Geometry: see drawing. Coordinates: mm, zero at the bounding-box minimum. A direction names the side the tool comes from. Give positions to 0.01 mm unless a question says otherwise; leave off trailing zeros. Order: outer loops, then holes, each group sorted by start corner. A loop starts at its lowest first (then second) coordinate and runs counter-clockwise, first axis right, second up. Notation, with made-up numbers: (55, 38) - (111, 38) arc R18 ccw to (111, 72) - close; hole circle Ø1 at (39, -27.75). An arc over 180 degrees is marked (long way). Write item = value, one per line. Start each with the question number.
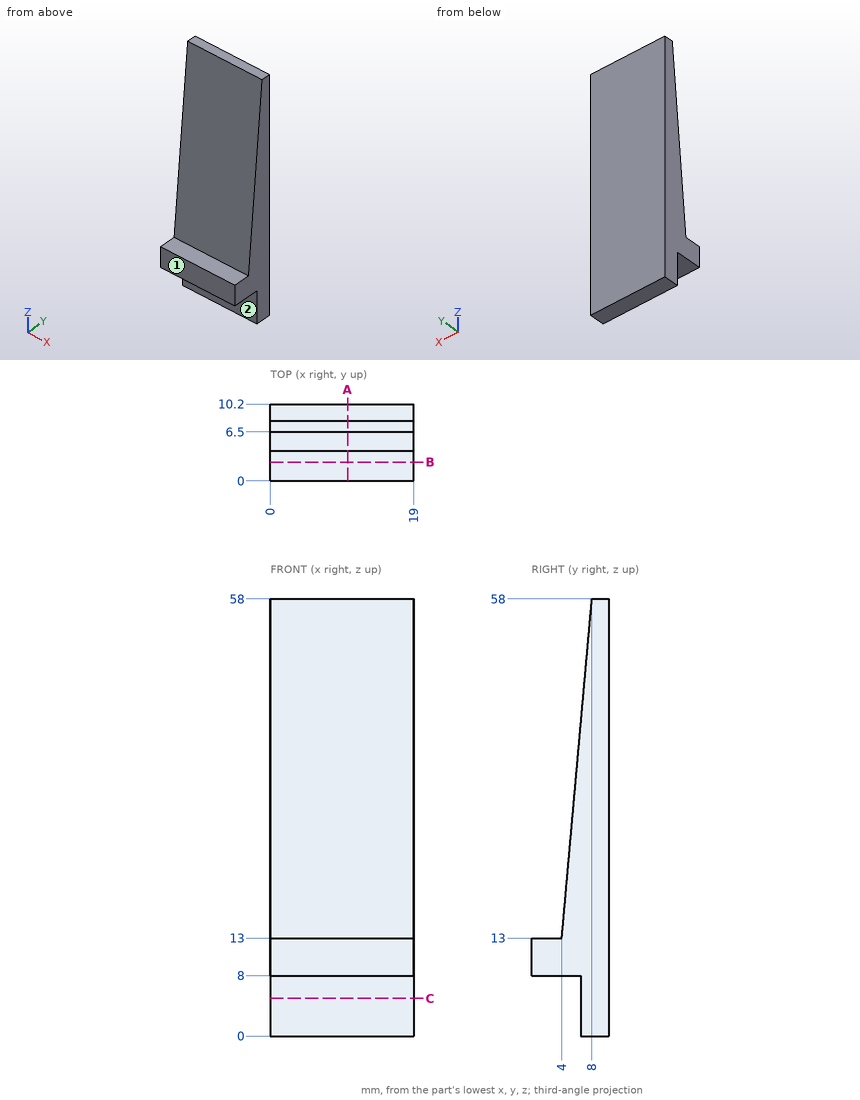
Q1. Material intervals for line 1 along Z through (x, y) = (13, 3.75); line 2 along Y through (x, z) = (2.25, 7); line 3 along Y through (x, z) = (7.25, 29.5), sorted ascending. Write a range as from..to.
Q2. Section A-A, the plane x = 10.25. Return the cut outline in (y, z).
Q3. Contact query for flat-ended pins moving along their axis: pin 1 (2 mm diameter, centred on y = 4, z = 39, fed in from -X); pin 2 (6 mm diameter, centred on x = 3.5, z = 42.5, fed in from -Y); pin 3 (4 mm diameter, centred on x = 6, z = 3.5, fed in from -Y); pin 4 (2 mm diameter, centred on x = 6, y = 2, fed in from +Z). Output: stop coordinate, or through.
Q4. Section B-B, the plane y = 2.5. Return the cut outline in (x, z), then the cut area to 3 significant figures.
Q5. Set-up query: the marked faces 1 and 2. Return all of +Z, -Z, +X, -X, +Y, -Y with unobstructed straight access to the full face (end or side cutting, diameter ignored); none if empty.
Q6. Section C-C, the plane z = 5. Return the cut outline in (x, y), then the cut area to 3 significant figures.
The answers:
q1.line_1 = 8..13
q1.line_2 = 6.5..10.2
q1.line_3 = 5.47..10.2
q2.outline = (0, 8) - (6.5, 8) - (6.5, 0) - (10.2, 0) - (10.2, 58) - (8, 58) - (4, 13) - (0, 13) - close
q3.pin_1 = through
q3.pin_2 = 6.36
q3.pin_3 = 6.5
q3.pin_4 = 13
q4.outline = (0, 8) - (19, 8) - (19, 13) - (0, 13) - close
q4.area = 95.0 mm²
q5.face_1 = +Z, -Z, +X, -X, -Y
q5.face_2 = -Z, +X, -X, -Y
q6.outline = (0, 6.5) - (19, 6.5) - (19, 10.2) - (0, 10.2) - close
q6.area = 70.3 mm²
